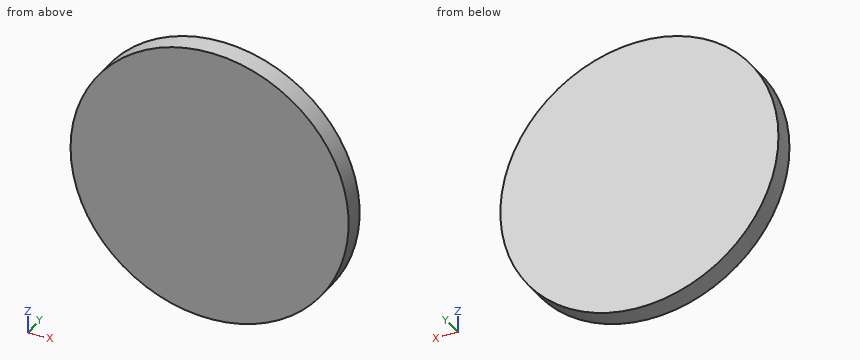
Autodesk Inventor part; units mm, degrees
ref_plane "YZ Plane" through (0, 0, 0) normal (1, 0, 0) x (0, 1, 0)
ref_plane "XZ Plane" through (0, 0, 0) normal (0, 1, 0) x (-1, 0, 0)
ref_plane "XY Plane" through (0, 0, 0) normal (0, 0, 1) x (1, 0, 0)
sketch "Skizze1" plane through (0, 0, 0) normal (0, 1, 0) x (-1, 0, 0)
  circle A0 centre (0, 0) radius 19.25
  circle A1 centre (0, 0) radius 19.75
  dimension "d0" = 38.5
  dimension "d1" = 0.5
extrude "Extrusion1" add sketch "Skizze1" along normal blind 3
sketch "Skizze2" plane through (0, 3, 0) normal (0, 1, 0) x (1, 0, 0)
  circle A0 centre (0, 0) radius 19.75
  line L0 (-10.9514, -0.5507) -> (-9.9514, -0.5507) construction
  circle A1 centre (0, 0) radius 19.75
  circle A2 centre (0, 0) radius 19.25
  arc A3 (-10.1928, -0.3825) -> (-10.1928, 0.3825) centre (-9.7907, 0) ccw
  circle A4 centre (0, 0) radius 19.25
  arc A5 (-9.9638, 0.85) -> (-9.7216, 0.5507) centre (-9.687, 0.8264) ccw
  arc A6 (-9.7216, -0.5507) -> (-9.9638, -0.85) centre (-9.687, -0.8264) ccw
  point P0 (-9.9865, 0.5193)
  point P1 (-9.9865, -0.5193)
  point P2 (-9.9865, 0.5193)
  point P3 (-9.9865, -0.5193)
  point P4 (-9.9638, 0.85)
  dimension "d9" = 1.11
  dimension "d10" = 0
  dimension "d11" = 1.7
  dimension "d12" = 0.85
  dimension "d14" = 9.7907
extrude "Extrusion2" add sketch "Skizze2" against normal up to surface (3 mm away) contours A2
pattern_circular "Runde Anordnung1" count 31 over 360 about axis through (0, 0, 0) along (0, 1, 0) of "Extrusion2"
equation "\"d12\" = 0.5 * d11"
properties part number "30_Cube_Z_Focus_MGN_NEMA_timingbelt_v3"
For this review, take the finished solid that the model builds, in its own axes (mm). Coordinates: 2 decimals unless noted, no trailing zeros. Loops run counter-clockwise (first coordinate to the right, second up) from the corner with the lowest first, then second, coordinate; pieces in that order, holes last. Notation, with made-up numbers: (45.25, 14) - (67.25, 14) arc R12 cw to (67.25, 30) - close; hole circle Ø1 at (62, 54.25). An arc over 180 degrees is marked (long way). Use a Markdown table: item, result. Add a question column.
Item 1: Insertion check: pin 1 Ø1 at (y, z) = (1, 3) entering from +X. The pin has a flat end and moves straight along its axis. Give the tip position at first contact, or say it passes through.
Item 2: We need section B-B (x = 13.5). Give the boundary of the cut face in (y, z), and give its area (3 significant figures).
Item 3: We need section A-A (y = 1.75). Give the boundary of the cut face in (x, z), and give its area (3 significant figures).
Item 4: We need section C-C (z = -12). Give the boundary of the cut face in (x, y).
Item 5: For line 1 (Z direction, x = -6.5, y = 2.45); line 2 (Z direction, x = -11, y = 0.1); line 3 (X direction, y = 1.5, z = -12), list the stretches that pass through material, from the lowest coordinate up.
Results list:
| question | item | result |
|---|---|---|
| 1 | pin 1 | stops at x = 19.59 |
| 2 | outline | (0, -14.42) - (3, -14.42) - (3, 14.42) - (0, 14.42) - close |
| 2 | area | 86.5 mm^2 |
| 3 | outline | circle Ø39.5 at (0, 0) |
| 3 | area | 1,230 mm^2 |
| 4 | outline | (-15.69, 0) - (15.69, 0) - (15.69, 3) - (-15.69, 3) - close |
| 5 | line 1 | z = -18.65 to 18.65 |
| 5 | line 2 | z = -16.4 to 16.4 |
| 5 | line 3 | x = -15.69 to 15.69 |
